Can you work these out from the model? Positions are in its coordinate system, mm. Face numbers are marked on the shaded views. A direction names the side the tool comes from. Round coordinates to 2 decimals unless told otherwise and drop trailing zeros. Order: outer loops, then holes, each group sorted by start corner. A loop starts at its lowest first (then second) coordinate and runs counter-clockwise, first axis right, second up.
Q1. If I drill on line 1 (Y direction, x = -5.5, z = 11); line 2 (Y direction, x = -9, z = 8.5); line 3 (Y direction, x = -13.5, z = -2) (3 decimals), over which ranges is the centre line in solid material (lowest first)?
Q2. If we section it at D-D (x = -16): Please give me the cut outline in (y, z) (3 decimals), plus the area to 3 significant figures.
Q3. Will these pins go through, and if not, where does the flat tip stop? P1, Ø1.2, axis at x = 9, z = -2.5, coming from the -Y side (3 decimals); P2, Ø2, axis at x = 1.5, z = 2, coming from the +Y side; P3, Ø14.5, axis at x = -8, y = 9.5, coming from the -Z side.
Q4. If we section it at C-C (z = 9.5): Please give me the cut outline in (x, y), plus the area to 3 significant figures.
Q5. If we section it at B-B (y = 14.5): Please give me the cut outline in (x, z).
Q6. If we section it at A-A (x = 0): Please give me the cut outline in (y, z) (3 decimals).
Q7. We'd pull the mould along Y, two halves only. Please class the marked faces 1, 2, 3 and 4: pulls with the +Y half, pulls with the -Y half, needs draft (parallel to the pull), parting line crosses it, or undercut.
Q8. For the marked faces 5, 6 and 7, which set-ups out of +Z, -Z, +X, -X, +Y, -Y let a thin tool reach every point of the face, with its end or its side?
from build123d import *

# Parameters (mm, degrees)
F0_R     = 20
F0_R_2   = 2.5
F1_DEPTH = 12
F3_DEPTH = 3.9
F5_DEPTH = 15.901
F7_DEPTH = 8


# Not quite as in the source:
# - after a boolean that leaves OpenCascade's solid faulty, fix() repairs it


with BuildPart() as f1:
    # F0 (on Top) → F1 (new body)
    with BuildSketch(Plane.XY):
        Circle(F0_R)
        with Locations((-9.8994949366, -9.8994949366)):
            Circle(F0_R_2, mode=Mode.SUBTRACT)
        with Locations((9.8994949366, -9.8994949366)):
            Circle(F0_R_2, mode=Mode.SUBTRACT)
        with Locations((-9.8994949366, 9.8994949366)):
            Circle(F0_R_2, mode=Mode.SUBTRACT)
        with Locations((9.8994949366, 9.8994949366)):
            Circle(F0_R_2, mode=Mode.SUBTRACT)
    extrude(amount=F1_DEPTH)

    # F2 (on face) → F3 (join)
    with BuildSketch(Plane(origin=(0, 0, 0), x_dir=(1, 0, 0), z_dir=(0, 0, -1))):
        with BuildLine():
            Line((19.9022454763, 1.975), (-19.9022454763, 1.975))
            ThreePointArc((-19.9022454763, 1.975), (-20, 0), (-19.9022454763, -1.975))
            Line((-19.9022454763, -1.975), (19.9022454763, -1.975))
            ThreePointArc((19.9022454763, -1.975), (19.9755464196, -0.9887088736), (20, 0))
            ThreePointArc((20, 0), (19.9755464196, 0.9887088736), (19.9022454763, 1.975))
        make_face()
    extrude(amount=F3_DEPTH)

    add(f1.part.fix(), mode=Mode.REPLACE)

    # F4 (on face) → F5 (cut, through all)
    with BuildSketch(Plane.XY.offset(12)):
        with BuildLine():
            Line((3.75, 17.5), (-3.75, 17.5))
            ThreePointArc((-3.75, 17.5), (-6.75, 14.5), (-3.75, 11.5))
            Line((-3.75, 11.5), (3.75, 11.5))
            ThreePointArc((3.75, 11.5), (6.75, 14.5), (3.75, 17.5))
        make_face()
        with BuildLine():
            ThreePointArc((3.75, -17.5), (6.75, -14.5), (3.75, -11.5))
            Line((3.75, -11.5), (-3.75, -11.5))
            ThreePointArc((-3.75, -11.5), (-6.75, -14.5), (-3.75, -17.5))
            Line((-3.75, -17.5), (3.75, -17.5))
        make_face()
    extrude(amount=-F5_DEPTH, mode=Mode.SUBTRACT)

    # F6 (on face) → F7 (cut)
    with BuildSketch(Plane.XY.offset(12)):
        with BuildLine():
            Line((3.75, 19), (-3.75, 19))
            ThreePointArc((-3.75, 19), (-8.25, 14.5), (-3.75, 10))
            Line((-3.75, 10), (3.75, 10))
            ThreePointArc((3.75, 10), (8.25, 14.5), (3.75, 19))
        make_face()
        with BuildLine():
            ThreePointArc((-3.75, 11.5), (-6.75, 14.5), (-3.75, 17.5))
            Line((-3.75, 17.5), (3.75, 17.5))
            ThreePointArc((3.75, 17.5), (6.75, 14.5), (3.75, 11.5))
            Line((3.75, 11.5), (-3.75, 11.5))
        make_face(mode=Mode.SUBTRACT)
        with BuildLine():
            ThreePointArc((3.75, -19), (8.25, -14.5), (3.75, -10))
            Line((3.75, -10), (-3.75, -10))
            ThreePointArc((-3.75, -10), (-8.25, -14.5), (-3.75, -19))
            Line((-3.75, -19), (3.75, -19))
        make_face()
        with BuildLine():
            ThreePointArc((3.75, -11.5), (6.75, -14.5), (3.75, -17.5))
            Line((3.75, -17.5), (-3.75, -17.5))
            ThreePointArc((-3.75, -17.5), (-6.75, -14.5), (-3.75, -11.5))
            Line((-3.75, -11.5), (3.75, -11.5))
        make_face(mode=Mode.SUBTRACT)
    extrude(amount=-F7_DEPTH, mode=Mode.SUBTRACT)


solid = f1.part
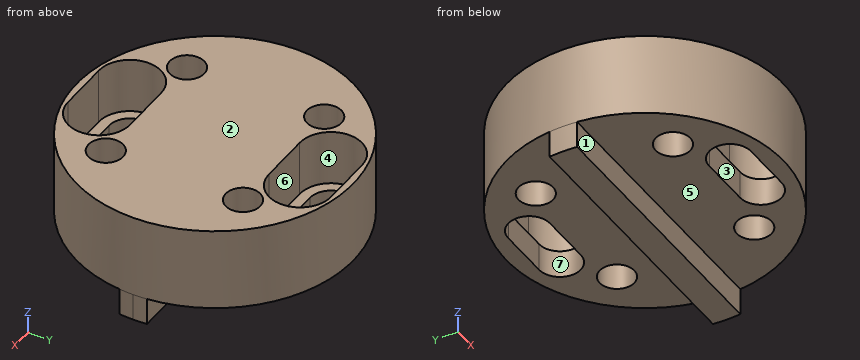
Solution:
1. line 1: y = -19.23 to -18.65, -10.35 to 10.35, 18.65 to 19.23
1. line 2: y = -17.86 to -12.23, -7.57 to 7.57, 12.23 to 17.86
1. line 3: y = -1.975 to 1.975
2. outline: (-12, 0) - (-1.975, 0) - (-1.975, -3.9) - (1.975, -3.9) - (1.975, 0) - (12, 0) - (12, 12) - (-12, 12) - close
2. area: 303 mm2
3. P1: stops at y = -1.975
3. P2: stops at y = 19.99
3. P3: stops at z = 0
4. outline: circle Ø40 at (0, 0); hole circle Ø5 at (-9.9, -9.9); hole circle Ø5 at (-9.9, 9.9); hole (-3.75, -19) - (3.75, -19) arc R4.5 ccw to (3.75, -10) - (-3.75, -10) arc R4.5 ccw to start; hole (-3.75, 10) - (3.75, 10) arc R4.5 ccw to (3.75, 19) - (-3.75, 19) arc R4.5 ccw to start; hole circle Ø5 at (9.9, -9.9); hole circle Ø5 at (9.9, 9.9)
4. area: 916 mm2
5. outline: (-13.77, 0) - (-6.75, 0) - (-6.75, 4) - (-8.25, 4) - (-8.25, 12) - (-13.77, 12) - close; (6.75, 0) - (13.77, 0) - (13.77, 12) - (8.25, 12) - (8.25, 4) - (6.75, 4) - close
6. outline: (-20, 0) - (-17.5, 0) - (-17.5, 4) - (-19, 4) - (-19, 12) - (-20, 12) - close; (-11.5, 0) - (-1.975, 0) - (-1.975, -3.9) - (1.975, -3.9) - (1.975, 0) - (11.5, 0) - (11.5, 4) - (10, 4) - (10, 12) - (-10, 12) - (-10, 4) - (-11.5, 4) - close; (17.5, 0) - (20, 0) - (20, 12) - (19, 12) - (19, 4) - (17.5, 4) - close
7. face 1: pulls with the -Y half
7. face 2: needs draft
7. face 3: undercut
7. face 4: undercut
8. face 5: -Z, +X, -X, -Y
8. face 6: +Z
8. face 7: +Z, -Z
